Input: part model. Units: mm. Frame: model coordinates. A direction names the side the tool comes from. Round coordinates to 2 decimals unless told otherwise and drop trailing zeros. Loops run counter-clockwise (first coordinate to the right, second up) from the corner with the lowest first, then second, coordinate; pieces in that order, holes last. Notation, with made-up numbers: (52.5, 73) - (95.5, 73) arc R17 ccw to (95.5, 85) - close; hole circle Ø9 at (63, 17.5). An arc over 180 degrees is marked (long way). One line per question, with ' | ' between items. Start each with the question number.
from build123d import *

# Parameters (mm, degrees)
F1_DEPTH = 15
F2_DEPTH = 7.5
F3_DEPTH = 7.5


with BuildPart() as f1:
    # F0 (on Front) → F1 (new body, symmetric)
    with BuildSketch(Plane.XZ):
        Polygon((0, 30), (0, 0), (40, 0), (40, 15), (30, 18.75), (10, 18.75), (10, 26.25), align=None)
        Polygon((10, 18.75), (30, 18.75), (20, 22.5), align=None)
        Polygon((20, 22.5), (10, 26.25), (10, 18.75), align=None)
    extrude(amount=F1_DEPTH, both=True)

    # F0 (on Front) → F2 (cut, symmetric)
    with BuildSketch(Plane.XZ):
        Polygon((20, 22.5), (10, 26.25), (10, 18.75), align=None)
    extrude(amount=F2_DEPTH, both=True, mode=Mode.SUBTRACT)

    # F0 (on Front) → F3 (join, symmetric)
    with BuildSketch(Plane.XZ):
        Polygon((20, 22.5), (30, 18.75), (30, 26.25), align=None)
    extrude(amount=F3_DEPTH, both=True)


solid = f1.part
(1) Section C-C, the plane x = 10.5. Output: boundary loops of the cut face in (y, z).
(2) Line query: line 1 along Z through (x, y) = (10, -9); line 2 along Y through (x, z) = (22, 22); line 3 along Z through (x, y) = (12, -4). Output: solid intervals per line, ascending. Write a range as from..to.
(3) Pull-direction query (Y, two-part tool) for faces 4 (the face through (14, 7.5, 23)), 5 (the face through (26, 7.5, 23)), 6 (the face through (0, 0, 15)); classes: released by +Y, released by -Y, zero draft, split by the parting line, or undercut.
(4) Section B-B, the plane z = 22. Output: boundary loops of the cut face in (x, y), plus the area to 3 significant figures.
(5) Reachability of faces 1 (the face through (30, 0, 22)), 2 (the face through (26, -7.5, 23)), 3 (the face through (14, -7.5, 23)) from +Z, -Z, +X, -X, +Y, -Y: full face, straight path, thin tool, end or side. Return the list, or none.
(6) Section A-A, the plane z = 25.25. Output: boundary loops of the cut face in (x, y).
(7) Pin query (flat end, axial travel): P1, Ø12, axis at y = -10, z = 25, coming from the +X side. Return the tip coordinate at first contact, or that it passes through.
(8) Section D-D, the plane z = 15.75. Output: boundary loops of the cut face in (x, y).
Derived:
1) outline: (-15, 0) - (15, 0) - (15, 26.06) - (7.5, 26.06) - (7.5, 18.94) - (-7.5, 18.94) - (-7.5, 26.06) - (-15, 26.06) - close
2) line 1: z = 0..26.25 | line 2: y = -7.5..7.5 | line 3: z = 0..19.5
3) face 4: undercut | face 5: released by +Y | face 6: zero draft
4) outline: (0, -15) - (21.33, -15) - (21.33, -7.5) - (30, -7.5) - (30, 7.5) - (21.33, 7.5) - (21.33, 15) - (0, 15) - close; hole (10, -7.5) - (18.67, -7.5) - (18.67, 7.5) - (10, 7.5) - close | area: 640 mm²
5) face 1: +Z, +X, +Y, -Y | face 2: +Z, +X, -Y | face 3: +Z
6) outline: (0, -15) - (12.67, -15) - (12.67, -7.5) - (10, -7.5) - (10, 7.5) - (12.67, 7.5) - (12.67, 15) - (0, 15) - close; (27.33, -7.5) - (30, -7.5) - (30, 7.5) - (27.33, 7.5) - close
7) P1: stops at x = 30
8) outline: (0, -15) - (38, -15) - (38, 15) - (0, 15) - close
